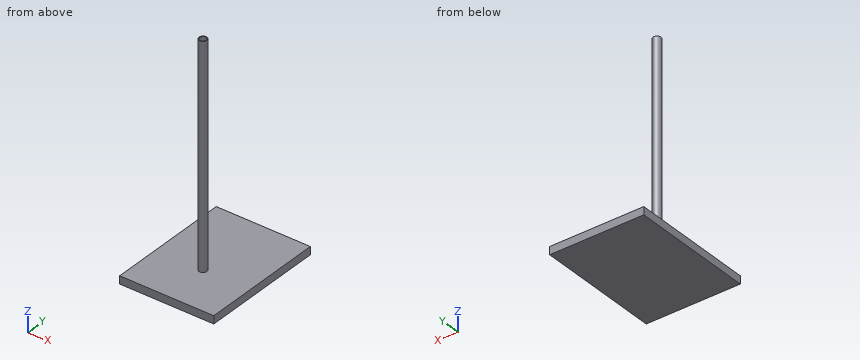
```python
from build123d import *

# Parameters (mm, degrees)
F0_W     = 300
F0_H     = 400
F1_DEPTH = 25
F2_R     = 12.5
F3_DEPTH = 700
F4_R     = 10
F5_DEPTH = 20


with BuildPart() as f1:
    # F0 (on Top) → F1 (new body)
    with BuildSketch(Plane.XY):
        with Locations((150, -200)):
            Rectangle(F0_W, F0_H)
    extrude(amount=F1_DEPTH)

    # F2 (on face) → F3 (join)
    with BuildSketch(Plane.XY.offset(25)):
        with Locations((150, -250)):
            Circle(F2_R)
    extrude(amount=F3_DEPTH)

    # F4 (on face) → F5 (cut)
    with BuildSketch(Plane.XY.offset(725)):
        with Locations((150, -250)):
            Circle(F4_R)
    extrude(amount=-F5_DEPTH, mode=Mode.SUBTRACT)


solid = f1.part
```
For this review, take the finished solid that the model builds, in its own axes (mm). Round coordinates to 2 decimals unless told otherwise and drop trailing zeros. Write each loop counter-clockwise with the first axis right and the second up, starting at its lowest first coordinate (ties: lowest second). Pieces come first, ordered by that corner, then holes. Notation, with made-up numbers: (-31.75, -29.5) - (-10.75, -29.5) arc R23 ccw to (-10.75, -2.5) - close; hole circle Ø8 at (11, 18). An arc over 180 degrees is marked (long way). Answer as a JSON object with one key per item and string values.
1. To check wall thickness, follow line 1 along Y through (x, z) = (150, 716.75); line 2 along Z through (x, y) = (216.5, -80). State the ranges of each line that lie inside material, in increasing order.
Response values:
{"line 1": "y = -262.5 to -260, -240 to -237.5", "line 2": "z = 0 to 25"}
2. We need section B-B on x = 150. Give the boundary of the cut face in (y, z).
Response values:
{"outline": "(-400, 0) - (0, 0) - (0, 25) - (-237.5, 25) - (-237.5, 725) - (-240, 725) - (-240, 705) - (-260, 705) - (-260, 725) - (-262.5, 725) - (-262.5, 25) - (-400, 25) - close"}
3. We need section D-D on x = 203. Give the boundary of the cut face in (y, z).
Response values:
{"outline": "(-400, 0) - (0, 0) - (0, 25) - (-400, 25) - close"}
4. For pin 1 Ø12 at (x, y) = (133.5, -325.5) entering from -Z; pin 2 Ø3 at (x, y) = (205.5, -73.5) entering from +Z; pin 3 Ø6 at (x, y) = (145, -245.5) entering from +Z, all flat-tipped, find the tip position at first contact; note any pin that passes through.
Response values:
{"pin 1": "stops at z = 0", "pin 2": "stops at z = 25", "pin 3": "stops at z = 705"}
5. We need section A-A on y = -250. Give the boundary of the cut face in (x, z), then the cut area to 3 significant figures.
Response values:
{"outline": "(0, 0) - (300, 0) - (300, 25) - (162.5, 25) - (162.5, 725) - (160, 725) - (160, 705) - (140, 705) - (140, 725) - (137.5, 725) - (137.5, 25) - (0, 25) - close", "area": "24,600 mm2"}
6. We need section C-C on z = 297. Give the boundary of the cut face in (x, y).
Response values:
{"outline": "circle Ø25 at (150, -250)"}
